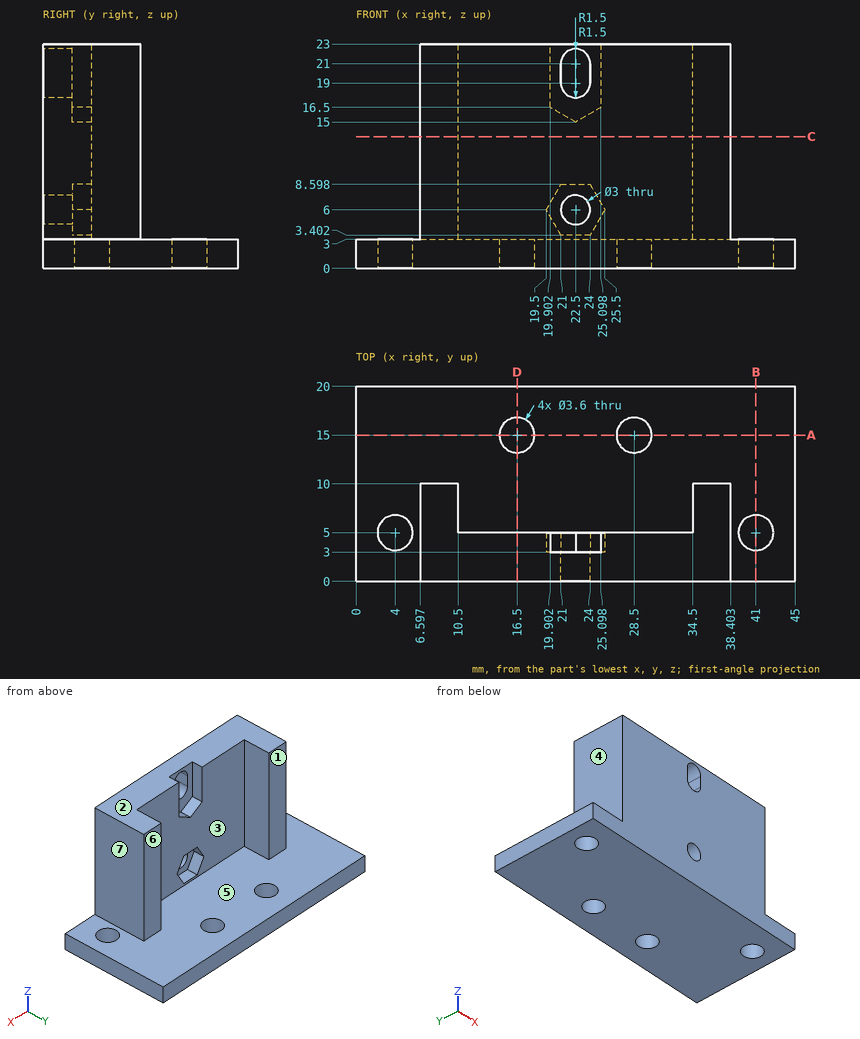
The figure shows three views and two pictorial views of one solid part (mm, origin at its lowest corner). Answer the questions. A direction names the side the tool comes from. Coordinates: 2 decimals unless noted, no trailing zeros. Write each loop counter-clockwise with the first axis right and the second up, starting at its lowest first coordinate (ties: lowest second). Pieces come first, ordered by that corner, then holes. Notation, with made-up numbers: M 62,-23.75 L 75,-23.75 A23 ccw 75,5.25 Z; hole C 81.5,17 d6. An arc over 180 degrees is marked long. Answer as CSV lines item,"result". Start each with the question number.
Item 1: Section C-C on z = 13.5 is taken. Write down the section's boundary in (x, y).
Item 2: Section A-A on y = 15 is taken. Write down the section's boundary in (x, z).
Item 3: Flat-ended cylindrical pins translate along their axes: P1, Ø6, axis at x = 38.5, y = 9.5, coming from the -Z side; P2, Ø4.5, axis at x = 41, y = 5, coming from the +Z side; P3, Ø5, axis at y = 7, z = 11.5, coming from the +X side; P4, Ø1.5, axis at y = 7, z = 16, coming from the -X side. Find the tip coordinate at first contact, or state that the pin passes through.
Item 4: Consider L1, parallel to Z at x = 22.5, y = 1.95; L2, parallel to X at y = 16.5, z = 2 (1 decimal); L3, parallel to Y at x = 16.5, z = 1.1. Determine where each line is inside the solid, lowest interval first.
Item 5: A tool of negligible diameter and unlimited length cuts with its end or side. For the marked faces 1, 2 and 3, from which of +Z, -Z, +X, -X, +Y, -Y can it reach the whole face along a straight path? Write none if from no direction.
Item 6: Determine the mould class of the marked faces 4, 5, 6 and 7 for opening direction X: released by +X, released by -X, zero draft, split by the parting line, or undercut.
Item 7: Section B-B on x = 41 is taken. Write down the section's boundary in (y, z).
Item 8: Section D-D on x = 16.5 is taken. Write down the section's boundary in (y, z), and give its area (3 significant figures).
Checks:
1,outline,"M 6.6,0 L 38.4,0 L 38.4,10 L 34.5,10 L 34.5,5 L 10.5,5 L 10.5,10 L 6.6,10 Z"
2,outline,"M 0,0 L 14.7,0 L 14.7,3 L 0,3 Z; M 18.3,0 L 26.7,0 L 26.7,3 L 18.3,3 Z; M 30.3,0 L 45,0 L 45,3 L 30.3,3 Z"
3,P1,"stops at z = 0"
3,P2,"stops at z = 3"
3,P3,"stops at x = 38.4"
3,P4,"stops at x = 6.6"
4,L1,"z = 0 to 4.5, 7.5 to 17.5, 22.5 to 23"
4,L2,"x = 0 to 15.5, 17.5 to 27.5, 29.5 to 45"
4,L3,"y = 0 to 13.2, 16.8 to 20"
5,face 1,"+Z, +X, -X, +Y"
5,face 2,"+Z, +X, -X, +Y, -Y"
5,face 3,"+Z, +Y"
6,face 4,"released by -X"
6,face 5,"undercut"
6,face 6,"zero draft"
6,face 7,"released by +X"
7,outline,"M 0,0 L 3.2,0 L 3.2,3 L 0,3 Z; M 6.8,0 L 20,0 L 20,3 L 6.8,3 Z"
8,outline,"M 0,0 L 13.2,0 L 13.2,3 L 5,3 L 5,23 L 0,23 Z; M 16.8,0 L 20,0 L 20,3 L 16.8,3 Z"
8,area,"149 mm²"
